Here's how the part is built. I have some questions about the finished solid (model axes, mm). Face numbers are marked on the shaded views. A direction names the side the tool comes from. Round coordinates to 2 decimals unless told otherwise and drop trailing zeros. Write each loop counter-clockwise with the first axis right and the second up, starting at its lowest first coordinate (ties: lowest second). Pieces come first, ordered by that corner, then holes. Notation, with made-up numbers: (-7.75, 0) - (9.25, 0) arc R11 cw to (9.25, 15) - close; hole circle Ø5 at (74, -25.5). An arc over 180 degrees is marked (long way). Write item = value, one per line. Start each with the question number.
Item 1: If I drill on line 1 along X through (y, z) = (23.25, 15); line 2 along Z through (x, y) = (-0.5, 23.5); line 3 along X through (y, z) = (5.4, 21.75), over which ranges is the centre line in solid material (lowest first)? Write a range as [from, to].
Item 2: Which directions (+Z, -Z, +X, -X, +Y, -Y) give clear straight access to the entire face, cutting with the end or side of a thin tool? Please do the marked faces 4 and 5.
Item 3: If we section it at C-C (z = -21.75): Please give me the cut outline in (x, y).
Item 4: If we section it at B-B (x = -23): Please give me the cut outline in (y, z), and give its area (3 significant figures).
Item 5: For P1, Ø1.2, axis at y = 26.5, z = -26, coming from the -X side; P2, Ø4.5, axis at x = -23, z = 21.75, coming from the -Y side; P3, Ø1.5, axis at x = 15.5, y = 27, coming from the -Z side, each with a flat end and sliding along its axis, tell me the tip position at first contact or that it passes through.
Item 6: Thinking about a two-plate mould opening in X: for the marked faces 1, 2 and 3, which applies, pulls with the +X half, pulls with the -X half, needs draft (parallel to the pull), parting line crosses it, or undercut?
Item 7: If we section it at A-A (y = 21.5): Please give me the cut outline in (x, z), and give its area (3 significant figures).
Item 8: If we section it at D-D (y = 2.5): Please give me the cut outline in (x, z).
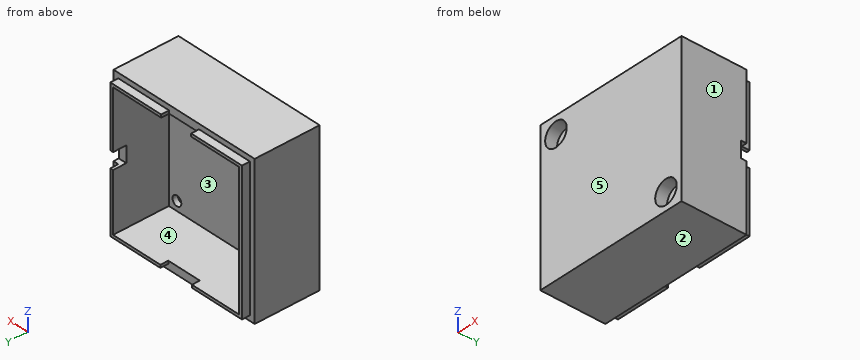
```python
from build123d import *

# Parameters (mm, degrees)
SKETCH1_W           = 59
SKETCH1_H           = 56.5
BOSS_EXTRUDE1_DEPTH = 6.5
SKETCH5_W           = 59
SKETCH5_H           = 56.5
SKETCH5_W_2         = 52.734513274
SKETCH5_H_2         = 50.5
BOSS_EXTRUDE2_DEPTH = 21.1
SKETCH6_W           = 59
SKETCH6_H           = 56.5
SKETCH6_W_2         = 55
SKETCH6_H_2         = 52.669491526
CUT_EXTRUDE2_DEPTH  = 3
SKETCH7_W           = 12.5
SKETCH7_H           = 2.169491525
SKETCH7_W_2         = 13.2
SKETCH7_H_2         = 3.830508475
SKETCH7_W_3         = 2.265486726
SKETCH7_H_3         = 6.1
CUT_EXTRUDE3_DEPTH  = 3
SKETCH9_W           = 3.132743363
SKETCH9_H           = 6.1
CUT_EXTRUDE5_DEPTH  = 2
SKETCH11_R          = 1.8526
CUT_EXTRUDE7_DEPTH  = 10
SKETCH12_R          = 4.5
CUT_EXTRUDE8_DEPTH  = 4.5


with BuildPart() as part:
    # Sketch1 → Boss-Extrude1 (new body)
    with BuildSketch(Plane(origin=(0, 0, 0), x_dir=(1, 0, 0), z_dir=(0, 1, 0))):
        Rectangle(SKETCH1_W, SKETCH1_H)
    extrude(amount=BOSS_EXTRUDE1_DEPTH)

    # Sketch5 → Boss-Extrude2 (add)
    with BuildSketch(Plane(origin=(0, 6.5, 0), x_dir=(1, 0, 0), z_dir=(0, 1, 0))):
        Rectangle(SKETCH5_W, SKETCH5_H)
        Rectangle(SKETCH5_W_2, SKETCH5_H_2, mode=Mode.SUBTRACT)
    extrude(amount=BOSS_EXTRUDE2_DEPTH)

    # Sketch6 → Cut-Extrude2 (cut)
    with BuildSketch(Plane(origin=(0, 27.6, 0), x_dir=(1, 0, 0), z_dir=(0, 1, 0))):
        Rectangle(SKETCH6_W, SKETCH6_H)
        Rectangle(SKETCH6_W_2, SKETCH6_H_2, mode=Mode.SUBTRACT)
    extrude(amount=-CUT_EXTRUDE2_DEPTH, mode=Mode.SUBTRACT)

    # Sketch7 → Cut-Extrude3 (cut)
    with BuildSketch(Plane(origin=(0, 27.6, 0), x_dir=(1, 0, 0), z_dir=(0, 1, 0))):
        with Locations((0, -26.334745762)):
            Rectangle(SKETCH7_W, SKETCH7_H)
        with Locations((0, 26.334745762)):
            Rectangle(SKETCH7_W_2, SKETCH7_H_2)
        with Locations((26.367256637, 0)):
            Rectangle(SKETCH7_W_3, SKETCH7_H_3)
    extrude(amount=-CUT_EXTRUDE3_DEPTH, mode=Mode.SUBTRACT)

    # Sketch9 → Cut-Extrude5 (cut)
    with BuildSketch(Plane(origin=(0, 24.6, 0), x_dir=(1, 0, 0), z_dir=(0, 1, 0))):
        with Locations((27.933628319, 0)):
            Rectangle(SKETCH9_W, SKETCH9_H)
    extrude(amount=-CUT_EXTRUDE5_DEPTH, mode=Mode.SUBTRACT)

    # Sketch11 → Cut-Extrude7 (cut)
    with BuildSketch(Plane(origin=(0, 0, 0), x_dir=(-1, 0, 0), z_dir=(0, -1, 0))):
        with Locations(Location((-23, 21.75, 0), (0, 0, 90))):
            Circle(SKETCH11_R)
        with Locations(Location((23, -21.75, 0), (0, 0, 90))):
            Circle(SKETCH11_R)
    extrude(amount=-CUT_EXTRUDE7_DEPTH, mode=Mode.SUBTRACT)

    # Sketch12 → Cut-Extrude8 (cut)
    with BuildSketch(Plane.XZ):
        with Locations(Location((-23, 21.75, 0), (0, 0, 270))):
            Circle(SKETCH12_R)
        with Locations(Location((23, -21.75, 0), (0, 0, 270))):
            Circle(SKETCH12_R)
    extrude(amount=-CUT_EXTRUDE8_DEPTH, mode=Mode.SUBTRACT)


solid = part.part
```
Reply:
q1.line_1 = [-29.5, -26.37], [26.37, 29.5]
q1.line_2 = [-28.25, -25.25], [25.25, 28.25]
q1.line_3 = [-29.5, -24.85], [-21.15, 29.5]
q2.face_4 = +Y
q2.face_5 = +Z, -Z, +X, -X, -Y
q3.outline = (-29.5, 0) - (18.5, 0) - (18.5, 4.5) - (21.15, 4.5) - (21.15, 6.5) - (-26.37, 6.5) - (-26.37, 27.6) - (-27.5, 27.6) - (-27.5, 24.6) - (-29.5, 24.6) - close; (24.85, 4.5) - (27.5, 4.5) - (27.5, 0) - (29.5, 0) - (29.5, 24.6) - (27.5, 24.6) - (27.5, 27.6) - (26.37, 27.6) - (26.37, 6.5) - (24.85, 6.5) - close
q4.outline = (0, -28.25) - (24.6, -28.25) - (24.6, -26.33) - (27.6, -26.33) - (27.6, -25.25) - (6.5, -25.25) - (6.5, 19.9) - (4.5, 19.9) - (4.5, 17.25) - (0, 17.25) - close; (0, 26.25) - (4.5, 26.25) - (4.5, 23.6) - (6.5, 23.6) - (6.5, 25.25) - (27.6, 25.25) - (27.6, 26.33) - (24.6, 26.33) - (24.6, 28.25) - (0, 28.25) - close
q4.area = 434 mm2
q5.P1 = -27.5
q5.P2 = 4.5
q5.P3 = -26.33
q6.face_1 = pulls with the +X half
q6.face_2 = needs draft
q6.face_3 = undercut
q7.outline = (-29.5, -28.25) - (29.5, -28.25) - (29.5, 28.25) - (-29.5, 28.25) - close; hole (-26.37, -25.25) - (26.37, -25.25) - (26.37, 25.25) - (-26.37, 25.25) - close
q7.area = 670 mm2
q8.outline = (-29.5, -28.25) - (29.5, -28.25) - (29.5, 28.25) - (-29.5, 28.25) - close; hole circle Ø9 at (-23, 21.75); hole circle Ø9 at (23, -21.75)
